from build123d import *

# Parameters (mm, degrees)
F0_W     = 230
F0_H     = 50
F1_DEPTH = 30
F2_R     = 5
F4_DEPTH = 76.7
F5_R     = 2.5
F6_DEPTH = 21


with BuildPart() as f1:
    # F0 (on Top) → F1 (new body)
    with BuildSketch(Plane.XY):
        Rectangle(F0_W, F0_H)
    extrude(amount=F1_DEPTH)

    # F2
    f2_edges = [f1.edges().sort_by_distance(p)[0] for p in [
        (115, -25, 15),
        (115, 25, 15),
        (115, 0, 30),
        (0, 25, 30),
        (0, -25, 30),
    ]]
    fillet(f2_edges, radius=F2_R)

    # F3 (on face) → F4 (cut)
    with BuildSketch(Plane.XZ.offset(25)):
        with BuildLine():
            ThreePointArc((-96.5, 15), (-99, 17.5), (-101.5, 15))
            ThreePointArc((-101.5, 15), (-99, 12.5), (-96.5, 15))
        make_face()
    extrude(amount=-F4_DEPTH, mode=Mode.SUBTRACT)

    # F5 (on face) → F6 (cut)
    with BuildSketch(Plane(origin=(0, 0, 0), x_dir=(1, 0, 0), z_dir=(0, 0, -1))):
        with Locations((93.5, 0)):
            Circle(F5_R)
    extrude(amount=-F6_DEPTH, mode=Mode.SUBTRACT)


solid = f1.part
The listing builds one solid part. Answer for the finished solid, in the listing's coordinates (mm). A direction names the side the tool comes from. Coordinates: 2 decimals unless noted, no trailing zeros. Write each loop counter-clockwise with the first axis right and the second up, starting at its lowest first coordinate (ties: lowest second). Pieces come first, ordered by that corner, then holes. Notation, with made-up numbers: (12, 41) - (65, 41) arc R13 ccw to (65, 65) - close; hole circle Ø4 at (68.5, -5.5). An arc over 180 degrees is marked (long way). Put each result on its own line as item: value.
1. A tool of negligible diameter and unlimited length cuts with its end or side. For faces 1 (the face through (93, 0, 21)), 2 (the face through (-4, 0, 30)), from which of +Z, -Z, +X, -X, +Y, -Y can it reach the whole face along a straight path? Write none if from no direction.
Answer sheet:
face 1: -Z
face 2: +Z, +X, -X, +Y, -Y
2. A flat-ended cylindrical pin translates along its axis: pin 1 Ø1.5 at (x, y) = (94, -1) entering from -Z. Find the tip coordinate at first contact, or state that the pin passes through.
Answer sheet:
pin 1: stops at z = 21
3. The part is cut by section A-A on z = 15. Give the vertices of the cut face in (x, y).
Answer sheet:
outline: (-115, -25) - (-101.5, -25) - (-101.5, 25) - (-115, 25) - close; (-96.5, -25) - (110, -25) arc R5 ccw to (115, -20) - (115, 20) arc R5 ccw to (110, 25) - (-96.5, 25) - close; hole circle Ø5 at (93.5, 0)
4. The part is cut by section C-C on x = 93.5. Give the vertices of the cut face in (y, z).
Answer sheet:
outline: (-25, 0) - (-2.5, 0) - (-2.5, 21) - (2.5, 21) - (2.5, 0) - (25, 0) - (25, 25) arc R5 ccw to (20, 30) - (-20, 30) arc R5 ccw to (-25, 25) - close
5. Find the intervals of material crossed by line 1 along Y through (x, z) = (93.5, 12.75); line 2 along Z through (x, y) = (-99, -2); line 3 along X through (y, z) = (13.5, 15), in increasing order. Write a range as from..to.
Answer sheet:
line 1: y = -25..-2.5, 2.5..25
line 2: z = 0..12.5, 17.5..30
line 3: x = -115..-101.5, -96.5..115
6. Determine the mould class of faces 3 (the face through (-97, -0.4, 16.5)), 4 (the face through (115, 0, 12)), 5 (the face through (-4, -25, 12)), 6 (the face through (91, 0, 10)) for opening direction X: pulls with the +X half, pulls with the -X half, needs draft (parallel to the pull), parting line crosses it, or undercut.
Answer sheet:
face 3: undercut
face 4: pulls with the +X half
face 5: needs draft
face 6: undercut
7. The part is cut by section B-B on y = 0. Give the vertices of the cut face in (x, z), plus the area to 3 significant figures.
Answer sheet:
outline: (-115, 0) - (91, 0) - (91, 21) - (96, 21) - (96, 0) - (115, 0) - (115, 25) arc R5 ccw to (110, 30) - (-115, 30) - close; hole circle Ø5 at (-99, 15)
area: 6,770 mm^2
